For this review, take the finished solid that the model builds, in its own axes (mm). Coordinates: 2 decimals unless noted, no trailing zeros. Write each loop counter-clockwise with the first axis right and the second up, starting at its lowest first coordinate (ties: lowest second). Pieces come first, ordered by that corner, then holes. Notation, with made-up numbers: (-23, 68.5) - (17, 68.5) arc R19 ccw to (17, 91.5) - close; hole circle Ø6 at (2.5, 70). An arc over 180 degrees is marked (long way). Write each question's results on one line, items separated by ' | '.
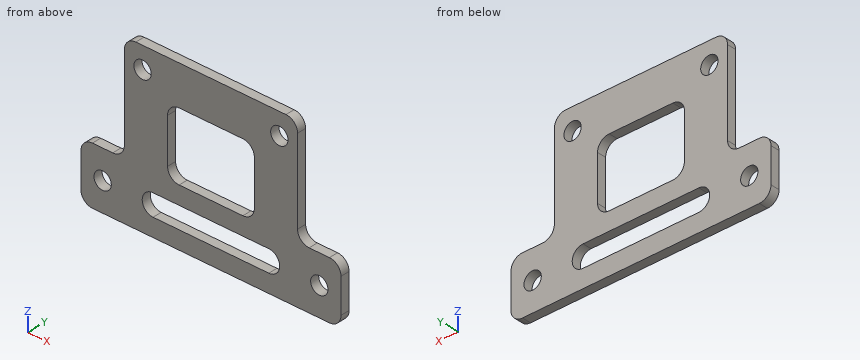
from build123d import *

# Parameters (mm, degrees)
SKETCH2_R           = 1.89865
SKETCH2_W           = 19.05
SKETCH2_H           = 15
BOSS_EXTRUDE1_DEPTH = 1.984375
FILLET1_R           = 2.54


with BuildPart() as part:
    # Sketch2 → Boss-Extrude1 (new body)
    with BuildSketch(Plane(origin=(0, 0, 0), x_dir=(1, 0, 0), z_dir=(0, 1, 0))):
        Polygon((0, 0), (0, 23.7625), (-9.525, 23.7625), (-9.525, 36.4625), (0, 36.4625), (38, 36.4625), (47.525, 36.4625), (47.525, 23.7625), (38, 23.7625), (38, 0), (27.055231083, 0), align=None)
        with Locations(Location((34, 4.7625, 0), (0, 0, 270))):
            Circle(SKETCH2_R, mode=Mode.SUBTRACT)
        with Locations(Location((4, 4.7625, 0), (0, 0, 270))):
            Circle(SKETCH2_R, mode=Mode.SUBTRACT)
        with Locations(Location((-4.7625, 30.1125, 0), (0, 0, 270))):
            Circle(SKETCH2_R, mode=Mode.SUBTRACT)
        with Locations(Location((42.7625, 30.1125, 0), (0, 0, 270))):
            Circle(SKETCH2_R, mode=Mode.SUBTRACT)
        with Locations((19, 16.2625)):
            Rectangle(SKETCH2_W, SKETCH2_H, mode=Mode.SUBTRACT)
        with BuildLine():
            Line((6.3, 32.49375), (31.7, 32.49375))
            ThreePointArc((31.7, 32.49375), (34.08125, 30.1125), (31.7, 27.73125))
            Line((31.7, 27.73125), (6.3, 27.73125))
            ThreePointArc((6.3, 27.73125), (3.91875, 30.1125), (6.3, 32.49375))
        make_face(mode=Mode.SUBTRACT)
    extrude(amount=BOSS_EXTRUDE1_DEPTH)

    # Fillet1
    fillet1_edges = [part.edges().sort_by_distance(p)[0] for p in [
        (0, 0.9921875, 0),
        (0, 0.9921875, -23.7625),
        (-9.525, 0.9921875, -23.7625),
        (-9.525, 0.9921875, -36.4625),
        (47.525, 0.9921875, -36.4625),
        (47.525, 0.9921875, -23.7625),
        (38, 0.9921875, -23.7625),
        (38, 0.9921875, 0),
        (28.525, 0.9921875, -8.7625),
        (28.525, 0.9921875, -23.7625),
        (9.475, 0.9921875, -23.7625),
        (9.475, 0.9921875, -8.7625),
    ]]
    fillet(fillet1_edges, radius=FILLET1_R)


solid = part.part
Q1. For pin 1 (0.6 mm diameter, centred on y = 1, z = -18, fed in from -X); pin 2 (3.5 mm diameter, centred on x = 4, z = -4.76, fed in from +Y); pin 3 (0.6 mm diameter, centred on x = -4, y = 1, fed in from +Z), all flat-tipped, find the tip position at first contact; note any pin that passes through.
Results found:
pin 1: x = 0 | pin 2: through | pin 3: z = -23.76
Q2. Take a section at C-C on x = 22. State the section outline as (y, z) points, plus the area to 3 significant figures.
Results found:
outline: (0, -36.46) - (1.98, -36.46) - (1.98, -32.49) - (0, -32.49) - close; (0, -27.73) - (1.98, -27.73) - (1.98, -23.76) - (0, -23.76) - close; (0, -8.76) - (1.98, -8.76) - (1.98, 0) - (0, 0) - close | area: 33.1 mm2
Q3. Wall thickness on line 1 along Z through (x, y) = (19, 1.05); line 2 along X through (y, z) = (0.6, -17) (3 decimals); line 3 along X through (y, z) = (1.7, -6.5): over which ranges is each line inside the solid? List them lowest first. Write a range as from..to.
Results found:
line 1: -36.46..-32.49, -27.73..-23.76, -8.76..0 | line 2: 0..9.475, 28.525..38 | line 3: 0..3.23, 4.77..33.23, 34.77..38
Q4. Take a section at B-B on x = 30. State the section outline as (y, z) points, plus the area to 3 significant figures.
Results found:
outline: (0, -36.46) - (1.98, -36.46) - (1.98, -32.49) - (0, -32.49) - close; (0, -27.73) - (1.98, -27.73) - (1.98, 0) - (0, 0) - close | area: 62.9 mm2
Q5. Take a section at D-D on y = 1.5. State how many separate pieces and enclosed holes the cut face has, plus the area to 3 significant figures.
Results found:
separate pieces: 1 | enclosed holes: 6 | area: 1,160 mm2
Q6. Take a section at A-A on z = -14.5. State the section outline as (x, y) points (3 decimals), plus the area to 3 significant figures.
Results found:
outline: (0, 0) - (9.475, 0) - (9.475, 1.984) - (0, 1.984) - close; (28.525, 0) - (38, 0) - (38, 1.984) - (28.525, 1.984) - close | area: 37.6 mm2
